from build123d import *

# Parameters (mm, degrees)
F0_R     = 2.5
F1_DEPTH = 1.5
F2_R     = 4.99999
F3_R     = 2.25
F4_DEPTH = 25
F5_W     = 4.6
F5_H     = 1.9
F5_W_2   = 9.2
F6_DEPTH = 25
F7_R     = 0.94999


# Not quite as in the source:
# - a fillet or chamfer is up to 0.001 mm smaller than in the source, because OpenCascade refuses the exact size


with BuildPart() as f1:
    # F0 (on Top) → F1 (new body)
    with BuildSketch(Plane.XY):
        Polygon((15, 47.5), (-15, 47.5), (-15, 27.5), (-25, 27.5), (-25, -27.5), (-15, -27.5), (-15, -47.5), (15, -47.5), (15, -27.5), (25, -27.5), (25, 27.5), (15, 27.5), align=None)
        with Locations((-7.5, -42.5)):
            Circle(F0_R, mode=Mode.SUBTRACT)
        with Locations((7.5, -42.5)):
            Circle(F0_R, mode=Mode.SUBTRACT)
        with Locations((-7.5, 42.5)):
            Circle(F0_R, mode=Mode.SUBTRACT)
        with Locations((7.5, 42.5)):
            Circle(F0_R, mode=Mode.SUBTRACT)
    extrude(amount=F1_DEPTH)

    # F2 (radius 5 in the source; OpenCascade refuses exactly that, so slightly less here)
    f2_edges = [f1.edges().sort_by_distance(p)[0] for p in [
        (15, 47.5, 0.75),
        (15, 27.5, 0.75),
        (25, 27.5, 0.75),
        (25, -27.5, 0.75),
        (15, -47.5, 0.75),
        (-15, 47.5, 0.75),
        (-15, 27.5, 0.75),
        (-25, 27.5, 0.75),
        (-25, -27.5, 0.75),
        (-15, -47.5, 0.75),
        (-15, -27.5, 0.75),
        (15, -27.5, 0.75),
    ]]
    fillet(f2_edges, radius=F2_R)

    # F3 (on face) → F4 (cut)
    with BuildSketch(Plane.XY.offset(1.5)):
        with Locations((0, 16.5)):
            Circle(F3_R)
        with Locations((0, 2)):
            Circle(F3_R)
        with Locations((15.75, -2.05)):
            Circle(F3_R)
        with Locations((-15.75, -2.05)):
            Circle(F3_R)
        with Locations((11.85, -13.95)):
            Circle(F3_R)
        with Locations((-11.85, -13.95)):
            Circle(F3_R)
    extrude(amount=-F4_DEPTH, mode=Mode.SUBTRACT)

    # F5 (on face) → F6 (cut)
    with BuildSketch(Plane.XY.offset(1.5)):
        with Locations((-2.3, 11.5)):
            Rectangle(F5_W, F5_H)
        with Locations((2.3, 11.5)):
            Rectangle(F5_W, F5_H)
        with Locations((0, -2.8)):
            Rectangle(F5_W_2, F5_H)
        Polygon((-11.7185466768, 4.111970797), (-13.524056425, 3.5202491148), (-10.6588777534, -5.2222191396), (-8.8533680052, -4.6304974575), align=None)
        Polygon((-9.624056425, -8.3797508852), (-6.7588777534, -17.1222191396), (-4.9533680052, -16.5304974575), (-7.8185466768, -7.788029203), align=None)
        Polygon((10.6588777534, -5.2222191396), (13.524056425, 3.5202491148), (11.7185466768, 4.111970797), (8.8533680052, -4.6304974575), align=None)
        Polygon((4.9533680052, -16.5304974575), (6.7588777534, -17.1222191396), (9.624056425, -8.3797508852), (7.8185466768, -7.788029203), align=None)
    extrude(amount=-F6_DEPTH, mode=Mode.SUBTRACT)

    # F7 (radius 0.95 in the source; OpenCascade refuses exactly that, so slightly less here)
    f7_edges = [f1.edges().sort_by_distance(p)[0] for p in [
        (13.524056, 3.520249, 0.75),
        (-8.853368, -4.630497, 0.75),
        (9.624056, -8.379751, 0.75),
        (-4.953368, -16.530497, 0.75),
        (-13.524056, 3.520249, 0.75),
        (-9.624056, -8.379751, 0.75),
        (8.853368, -4.630497, 0.75),
        (4.953368, -16.530497, 0.75),
        (-4.6, 12.45, 0.75),
        (-4.6, -1.85, 0.75),
        (-11.718547, 4.111971, 0.75),
        (11.718547, 4.111971, 0.75),
        (-7.818547, -7.788029, 0.75),
        (7.818547, -7.788029, 0.75),
        (4.6, -1.85, 0.75),
        (4.6, 12.45, 0.75),
        (10.658878, -5.222219, 0.75),
        (-10.658878, -5.222219, 0.75),
        (-4.6, -3.75, 0.75),
        (-4.6, 10.55, 0.75),
        (4.6, 10.55, 0.75),
        (4.6, -3.75, 0.75),
        (-6.758878, -17.122219, 0.75),
        (6.758878, -17.122219, 0.75),
    ]]
    fillet(f7_edges, radius=F7_R)


solid = f1.part
The model under review builds one solid part; all positions refer to its coordinate system, in mm. A direction names the side the tool comes from. Round coordinates to 2 decimals unless told otherwise and drop trailing zeros. Loops run counter-clockwise (first coordinate to the right, second up) from the corner with the lowest first, then second, coordinate; pieces in that order, holes last. Notation, with made-up numbers: (71.5, 45.5) -> (93.5, 45.5) arc R8 cw to (93.5, 58.5) -> close; hole circle Ø6 at (12, -19). An arc over 180 degrees is marked (long way). Write item = value, one per line. Start each with the question number.
Item 1: Mouldability with a two-part tool opening along X and no side actions: class faces 1 (the cylindrical face through (-16.5, -28.93, 0.76)), 2 (the cylindrical face through (6.96, 40.06, 0.74)), 3 (the flat face through (-6, 1, 1.5)) as released by +X, released by -X, zero draft, split by the parting line, or undercut.
Item 2: Take a section at B-B on x = -16.5. Give the boundary of the cut face in (y, z).
Item 3: Insertion check: pin 1 (0.8 mm diameter, centred on y = 36, z = 1, fed in from +X). The pin has a flat end and moves straight along its axis. Give the tip position at first contact, or say it passes through.
Item 4: To check wall thickness, follow L1, parallel to Y at x = -3, z = 1.1; L2, parallel to X at y = -32.5, z = 0.2; L3, parallel to Y at x = 15.75, z = 1. State the ranges of each line that lie inside material, in increasing order.
Item 5: Take a section at C-C on y = -13.95. Give the boundary of the cut face in (x, z).
Item 6: Take a section at A-A on y = 16.5. Give the boundary of the cut face in (x, z), plus the area to 4 significant figures.
Item 7: Take a section at D-D on z = 0.6. Count the separate pieces of the cut face and the enclosed holes in it, plus the area to 3 significant figures.
Item 8: For faces 4 (the flat face through (-6.37, -12.21, 0.76)), 5 (the cylindrical face through (23.5, 26.07, 0.76)), list the 3-axis set-ups (+Z, -Z, +X, -X, +Y, -Y) from which the entire face can be reached by the end or side of a thin tool; tool diameter is ignored.
Result:
q1.face_1 = released by -X
q1.face_2 = undercut
q1.face_3 = zero draft
q2.outline = (-28.93, 0) -> (-4.17, 0) -> (-4.17, 1.5) -> (-28.93, 1.5) -> close; (0.07, 0) -> (28.93, 0) -> (28.93, 1.5) -> (0.07, 1.5) -> close
q3.pin_1 = 15
q4.L1 = -47.5 to -3.75, -1.85 to 10.55, 12.45 to 47.5
q4.L2 = -15 to 15
q4.L3 = -29.87 to -4.3, 0.2 to 29.87
q5.outline = (-25, 0) -> (-14.1, 0) -> (-14.1, 1.5) -> (-25, 1.5) -> close; (-9.6, 0) -> (-7.8, 0) -> (-7.8, 1.5) -> (-9.6, 1.5) -> close; (-5.8, 0) -> (5.8, 0) -> (5.8, 1.5) -> (-5.8, 1.5) -> close; (7.8, 0) -> (9.6, 0) -> (9.6, 1.5) -> (7.8, 1.5) -> close; (14.1, 0) -> (25, 0) -> (25, 1.5) -> (14.1, 1.5) -> close
q6.outline = (-25, 0) -> (-2.25, 0) -> (-2.25, 1.5) -> (-25, 1.5) -> close; (2.25, 0) -> (25, 0) -> (25, 1.5) -> (2.25, 1.5) -> close
q6.area = 68.25 mm²
q7.separate_pieces = 1
q7.enclosed_holes = 16
q7.area = 3,650 mm²
q8.face_4 = +Z, -Z
q8.face_5 = +Z, -Z, +X, +Y
